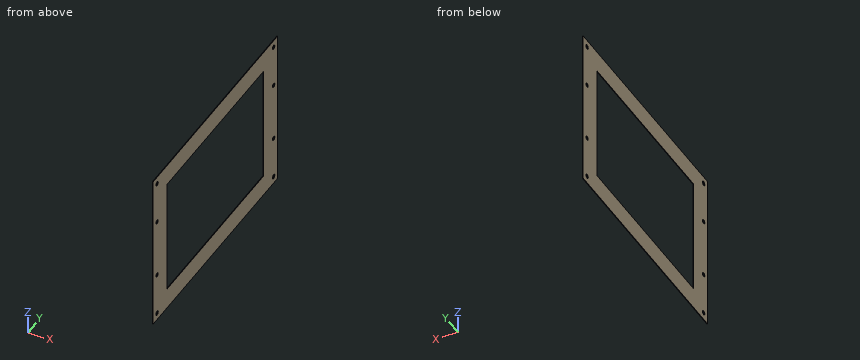
from build123d import *

# Parameters (mm, degrees)
SKETCH1_W           = 321
SKETCH1_H           = 220
BOSS_EXTRUDE1_DEPTH = 1
SKETCH2_R           = 3
CUT_EXTRUDE1_DEPTH  = 195.579675198
SKETCH3_W           = 249
SKETCH3_H           = 162
CUT_EXTRUDE2_DEPTH  = 195.579675198
SKETCH4_R           = 3
CUT_EXTRUDE3_DEPTH  = 195.579675198


with BuildPart() as part:
    # Sketch1 → Boss-Extrude1 (new body)
    with BuildSketch(Plane.YZ):
        Rectangle(SKETCH1_W, SKETCH1_H)
    extrude(amount=BOSS_EXTRUDE1_DEPTH)

    # Sketch2 → Cut-Extrude1 (cut, through all)
    with BuildSketch(Plane.YZ.offset(1)):
        with Locations(Location((-150.5, 100, 0), (0, 0, 270))):
            Circle(SKETCH2_R)
        with Locations(Location((150.5, 100, 0), (0, 0, 90))):
            Circle(SKETCH2_R)
        with Locations(Location((-150.5, -100, 0), (0, 0, 90))):
            Circle(SKETCH2_R)
        with Locations(Location((150.5, -100, 0), (0, 0, 270))):
            Circle(SKETCH2_R)
    extrude(amount=-CUT_EXTRUDE1_DEPTH, mode=Mode.SUBTRACT)

    # Sketch3 → Cut-Extrude2 (cut, through all)
    with BuildSketch(Plane.YZ.offset(1)):
        Rectangle(SKETCH3_W, SKETCH3_H)
    extrude(amount=-CUT_EXTRUDE2_DEPTH, mode=Mode.SUBTRACT)

    # Sketch4 → Cut-Extrude3 (cut, through all)
    with BuildSketch(Plane.YZ.offset(1)):
        with Locations(Location((-150.5, 41, 0), (0, 0, 270))):
            Circle(SKETCH4_R)
        with Locations(Location((150.5, 41, 0), (0, 0, 90))):
            Circle(SKETCH4_R)
        with Locations(Location((-150.5, -41, 0), (0, 0, 90))):
            Circle(SKETCH4_R)
        with Locations(Location((150.5, -41, 0), (0, 0, 270))):
            Circle(SKETCH4_R)
    extrude(amount=-CUT_EXTRUDE3_DEPTH, mode=Mode.SUBTRACT)


solid = part.part
Source: CAD feature listing. Evaluate the final solid. Frame: model axes, mm. Coordinates: 2 decimals unless noted, no trailing zeros. Loops run counter-clockwise (first coordinate to the right, second up) from the corner with the lowest first, then second, coordinate; pieces in that order, holes last. Notation, with made-up numbers: (47.25, 15) - (63.25, 15) arc R27 ccw to (63.25, 35) - close; hole circle Ø7 at (39.5, 86.5). An arc over 180 degrees is marked (long way). One line per item, written item: value. Start each with the question number.
1. Section C-C (x = 0.35). State how many separate pieces and enclosed holes the cut face has, and give its area (3 significant figures).
2. Ray query, L1, parallel to Y at x = 0.7, z = 41; L2, parallel to Z at x = 0.65, y = -150.5; L3, parallel to Y at x = 0.3, z = -65. Return the intervals inside material, ascending.
3. Section A-A (z = -16.5). Return the cut outline in (x, y).
4. Section B-B (y = 89). Return the cut outline in (x, z), and give its area (3 significant figures).
5. Contact query for a flat-ended pin moving along its axis: P1, Ø5.5, axis at y = -150.5, z = -100, coming from the +X side. Output: stop coordinate, or through.
Verdict:
1. separate pieces: 1
1. enclosed holes: 9
1. area: 30,100 mm2
2. L1: y = -160.5 to -153.5, -147.5 to -124.5, 124.5 to 147.5, 153.5 to 160.5
2. L2: z = -110 to -103, -97 to -44, -38 to 38, 44 to 97, 103 to 110
2. L3: y = -160.5 to -124.5, 124.5 to 160.5
3. outline: (0, -160.5) - (1, -160.5) - (1, -124.5) - (0, -124.5) - close; (0, 124.5) - (1, 124.5) - (1, 160.5) - (0, 160.5) - close
4. outline: (0, -110) - (1, -110) - (1, -81) - (0, -81) - close; (0, 81) - (1, 81) - (1, 110) - (0, 110) - close
4. area: 58.0 mm2
5. P1: passes through
